from build123d import *

# Parameters (mm, degrees)
EXTRUDE_THIN1_DEPTH = 9.62000108
CUT_EXTRUDE1_DEPTH  = 80.723760299
FILLET1_R           = 6.35
SKETCH4_W           = 2.00000108
SKETCH4_H           = 1.27
BOSS_EXTRUDE1_DEPTH = 2.54
SCALE1_SCALE        = 2.54


with BuildPart() as part:
    # Sketch2 → Extrude-Thin1 (new, symmetric)
    with BuildSketch(Plane(origin=(0, 0, 0), x_dir=(1, 0, 0), z_dir=(0, 1, 0))):
        Polygon((0, 0), (19.24000216, 0), (39.56000216, 12.7), (77.66000216, 12.7), (77.66000216, 10.16), (40.288464575, 10.16), (19.968464575, -2.54), (0, -2.54), align=None)
    extrude(amount=EXTRUDE_THIN1_DEPTH, both=True)

    # Sketch3 → Cut-Extrude1 (cut, through all)
    with BuildSketch(Plane.XY.offset(2.54)):
        with BuildLine():
            Line((6.35, 8.37540108), (12.91540216, 8.37540108))
            ThreePointArc((12.91540216, 8.37540108), (16.507504608, 6.887503528), (17.99540216, 3.29540108))
            Line((17.99540216, 3.29540108), (17.99540216, -3.27000108))
            ThreePointArc((17.99540216, -3.27000108), (16.507504608, -6.862103528), (12.91540216, -8.35000108))
            Line((12.91540216, -8.35000108), (6.35, -8.35000108))
            ThreePointArc((6.35, -8.35000108), (2.757897552, -6.862103528), (1.27, -3.27000108))
            Line((1.27, -3.27000108), (1.27, 3.29540108))
            ThreePointArc((1.27, 3.29540108), (2.757897552, 6.887503528), (6.35, 8.37540108))
        make_face()
    extrude(amount=-CUT_EXTRUDE1_DEPTH, mode=Mode.SUBTRACT)

    # Fillet1
    fillet1_edges = [part.edges().sort_by_distance(p)[0] for p in [
        (0, 9.62000108, 1.27),
        (0, -9.62000108, 1.27),
        (77.66000216, 9.62000108, -11.43),
        (77.66000216, -9.62000108, -11.43),
    ]]
    fillet(fillet1_edges, radius=FILLET1_R)

    # Sketch4 → Boss-Extrude1 (add)
    with BuildSketch(Plane.XY.offset(2.54)):
        with Locations((8.63270054, -8.98500108)):
            Rectangle(SKETCH4_W, SKETCH4_H)
    extrude(amount=BOSS_EXTRUDE1_DEPTH)


with BuildPart() as part_1:
    # Scale1: scaled about (44.171942925, -0.020471779, -8.083535651)
    add(part.part.scale(SCALE1_SCALE).moved(Location((-68.024792105, 0.03152654, 12.448644903))))


solid = part_1.part
Input: part model. Units: mm. Frame: model coordinates. A direction names the side the tool comes from. Coordinates: 2 decimals unless noted, no trailing zeros. Loops run counter-clockwise (first coordinate to the right, second up) from the corner with the lowest first, then second, coordinate; pieces in that order, holes last.
Q1. Draft query along X for faces 4 (the face through (-60.919, -17.498, 15.72)), 5 (the face through (-48.638, -23, 22)), 6 (the face through (80, 0, -19.809)). Return one class per face: +X half, -X half, draft (parallel to the pull), parting line (faces both ways), or undercut.
Q2. Cut plane C-C (y = 15.5). Output: boundary loops of the cut face in (x, z).
Q3. Contact query for flat-ended pins moving along their axis: pin 1 (12 mm diameter, centred on y = 8.5, z = -4, fed in from -X); pin 2 (1 mm diameter, centred on y = 19.5, z = 12, fed in from +X); pin 3 (8 mm diameter, centred on y = 17, z = -2.5, fed in from -X). Output: stop coordinate, or through.
Q4. Material intervals for line 1 (Z direction, x = 97, y = -11.5); line 2 (Y direction, x = -31, z = 17.5); line 3 (X direction, y = 15.5, z = 15.5), sorted ascending.
Q5. Cut plane A-A (y = 5). Output: boundary loops of the cut face in (x, z), then the cut area to 3 significant figures.
Q6. Set-up query: faces 1 (the face through (-22, 0, 12.449)), 2 (the face through (-22.316, 0, 16)), 3 (the face through (-43.558, -23, 22)). Return all of +Z, -Z, +X, -X, +Y, -Y with unobstructed straight access to the full face (end or side cutting, diameter ignored); none if empty.
Q7. Cut plane B-B (x = 108). Output: boundary loops of the cut face in (y, z), then the cut area to 3 significant figures.
Q8. Cut plane D-D (z = -4). Output: boundary loops of the cut face in (x, y).
Working result:
1. face 4: undercut
1. face 5: -X half
1. face 6: draft
2. outline: (-66.35, 12.45) - (-62.67, 12.45) - (-62.67, 18.9) - (-66.35, 18.9) - close; (-24.44, 12.45) - (-19.16, 12.45) - (32.46, -19.81) - (127.55, -19.81) - (127.55, -13.36) - (34.31, -13.36) - (-17.3, 18.9) - (-24.44, 18.9) - close
3. pin 1: stops at x = -2.44
3. pin 2: stops at x = -5.46
3. pin 3: stops at x = -1.64
4. line 1: z = -19.81 to -13.36
4. line 2: y = -24.4 to -20.47, 20.6 to 24.47
4. line 3: x = -66.35 to -62.67, -24.44 to -11.86
5. outline: (-68.02, 12.45) - (-64.8, 12.45) - (-64.8, 18.9) - (-68.02, 18.9) - close; (-22.32, 12.45) - (-19.16, 12.45) - (32.46, -19.81) - (129.23, -19.81) - (129.23, -13.36) - (34.31, -13.36) - (-17.3, 18.9) - (-22.32, 18.9) - close
5. area: 1,060 mm2
6. face 1: -Z, -X, +Y, -Y
6. face 2: +Z, -Z
6. face 3: +Z, +X, +Y, -Y
7. outline: (-24.4, -19.81) - (24.47, -19.81) - (24.47, -13.36) - (-24.4, -13.36) - close
7. area: 315 mm2
8. outline: (7.16, -24.4) - (19.34, -24.4) - (19.34, 24.47) - (7.16, 24.47) - close
